Verification items for the finished model (mm, model axes). A direction names the side the tool comes from. Coordinates: 2 decimals unless noted, no trailing zeros. Order: outer loops, then holes, each group sorted by start corner. A loop starts at its lowest first (then second) coordinate and runs counter-clockwise, first axis right, second up.
Q1. Set-up check for faces 5 (the cylindrical face through (9.392, 2.714, -9.769)), 6 (the cylindrical face through (9.66, 3.62, -8.88)): record each of +Z, -Z, +X, -X, +Y, -Y from which the full face is reachable in a straight line by a thin tool's end or side.
Q2. Cross-section at C-C, the plane x = 15. Record the boundary of the cut face in (y, z).
Q3. Cross-section at B-B, the plane y = 3.25. Record the boundary of the cut face in (x, z), and give its area (3 significant figures).
Q4. Draft check along X on faces 1 (the cylindrical face through (29.036, 2.931, 6.261)), 2 (the cylindrical face through (-9.08, 3.82, 6.26)), 3 (the cylindrical face through (27.93, 3.62, 6.26)), 4 (the flat face through (9.4, 12.7, -13.5)). Enter one of: pulls with the +X half, pulls with the -X half, needs draft (parallel to the pull), parting line crosses it, or undercut.
Q5. Depth check by flat-ended pin: P1, Ø5, axis at x = 0, y = 3, coming from the -Z side; P2, Ø4, axis at x = -9, z = -2.5, coming from the -Y side; P3, Ø6.5, axis at x = 8.5, z = 8.5, coming from the +Y side. Enter the tip coordinate at first touch or a pass-through.
Q6. Cross-section at A-A, the plane z = 2. Record the boundary of the cut face in (x, y), and give its area (3 significant figures).
Q7. Thickness scan on line 1 (X direction, y = 6, z = 10.5); line 2 (X direction, y = 7.25, z = 4); line 3 (Y direction, x = 19, z = 3). Record the ranges inside material, lowest first.
Q8. Cross-section at D-D, the plane y = 9. Record the boundary of the cut face in (x, z), and give its area (3 significant figures).
from build123d import *

# Parameters (mm, degrees)
REVOLVE_THIN1_ANGLE = 90
EXTRUDE_THIN1_DEPTH = 12.7


with BuildPart() as part:
    # Sketch1 → Revolve-Thin1 (revolve)
    with BuildSketch(Plane.XY):
        with BuildLine():
            ThreePointArc((-12.7, 12.7), (-8.980256121, 3.719743879), (0, 0))
            Line((0, 0), (19.05, 0))
            ThreePointArc((19.05, 0), (28.030256121, 3.719743879), (31.75, 12.7))
            Line((31.75, 12.7), (33.02, 12.7))
            ThreePointArc((33.02, 12.7), (28.928281733, 2.821718267), (19.05, -1.27))
            Line((19.05, -1.27), (0, -1.27))
            ThreePointArc((0, -1.27), (-9.878281733, 2.821718267), (-13.97, 12.7))
            Line((-13.97, 12.7), (-12.7, 12.7))
        make_face()
    revolve(axis=Axis((-12.7, 12.7, 0), (1, 0, 0)), revolution_arc=REVOLVE_THIN1_ANGLE)

    # Sketch1<2> → Extrude-Thin1 (add)
    with BuildSketch(Plane.XY):
        with BuildLine():
            ThreePointArc((-12.7, 12.7), (-8.980256121, 3.719743879), (0, 0))
            Line((0, 0), (19.05, 0))
            ThreePointArc((19.05, 0), (28.030256121, 3.719743879), (31.75, 12.7))
            Line((31.75, 12.7), (33.02, 12.7))
            ThreePointArc((33.02, 12.7), (28.928281733, 2.821718267), (19.05, -1.27))
            Line((19.05, -1.27), (0, -1.27))
            ThreePointArc((0, -1.27), (-9.878281733, 2.821718267), (-13.97, 12.7))
            Line((-13.97, 12.7), (-12.7, 12.7))
        make_face()
    extrude(amount=EXTRUDE_THIN1_DEPTH)


solid = part.part
Check values:
1. face 5: -Z, +X, -X, -Y
1. face 6: +Z, +Y
2. outline: (-1.27, 0) arc R13.97 ccw to (12.7, -13.97) - (12.7, -12.7) arc R12.7 cw to (0, 0) - (0, 12.7) - (-1.27, 12.7) - close
3. outline: (-10.29, 0) arc R10.29 ccw to (0, -10.29) - (19.05, -10.29) arc R10.29 ccw to (29.34, 0) - (29.34, 12.7) - (27.53, 12.7) - (27.53, 0) arc R8.48 cw to (19.05, -8.48) - (0, -8.48) arc R8.48 cw to (-8.48, 0) - (-8.48, 12.7) - (-10.29, 12.7) - close
3. area: 133 mm2
4. face 1: pulls with the +X half
4. face 2: undercut
4. face 3: undercut
4. face 4: needs draft
5. P1: stops at z = -11.97
5. P2: stops at y = 0.81
5. P3: stops at y = 0
6. outline: (-13.97, 12.7) arc R13.97 ccw to (0, -1.27) - (19.05, -1.27) arc R13.97 ccw to (33.02, 12.7) - (31.75, 12.7) arc R12.7 cw to (19.05, 0) - (0, 0) arc R12.7 cw to (-12.7, 12.7) - close
6. area: 77.4 mm2
7. line 1: x = -12.26 to -10.79, 29.84 to 31.31
7. line 2: x = -12.86 to -11.47, 30.52 to 31.91
7. line 3: y = -1.27 to 0
8. outline: (-13.47, 0) arc R13.47 ccw to (0, -13.47) - (19.05, -13.47) arc R13.47 ccw to (32.52, 0) - (32.52, 12.7) - (31.2, 12.7) - (31.2, 0) arc R12.15 cw to (19.05, -12.15) - (0, -12.15) arc R12.15 cw to (-12.15, 0) - (-12.15, 12.7) - (-13.47, 12.7) - close
8. area: 112 mm2
